Geometry: final body of the model. Coordinates: model frame, mm. A direction names the side the tool comes from. Coordinates: 2 decimals unless noted, no trailing zeros. Answer as a JSON object with one key per item and string values. Group by question number.
Item 1: Set-up query: faces 1 (the cylindrical face through (2.75, -62.44, -10.51)), 2 (the flat face through (-46, 37, -7.3)). Return all of +Z, -Z, +X, -X, +Y, -Y with unobstructed straight access to the full face (end or side cutting, diameter ignored); none if empty.
Item 2: Line query: line 1 along Z through (x, y) = (52.5, 26); line 2 along X through (y, z) = (0, -2); line 3 along X through (y, z) = (0, 0). Output: solid intervals per line, ascending. Write a range as from..to.
Item 3: Mould query, pull axis Z, two halves, no side actions, for faces 3 (the cylindrical face through (-57.11, -12.68, -4.22)), 4 (the cylindrical face through (-57.11, -12.68, 4.18)), 5 (the flat face through (-32, -47, -11.5)), 6 (the cylindrical face through (2.75, -62.44, 6.29)). Classes: pulls with the +Z half, pulls with the -Z half, needs draft (parallel to the pull), parting line crosses it, or undercut.
Item 4: First-contact query: pin 1 Ø1 at (y, z) = (-31.5, 6.5) entering from -X; pin 2 Ø5 at (y, z) = (4, 4.5) entering from -X; pin 3 Ø6 at (x, z) = (19, 0) entering from +Y. Flat tips, straight axial feed; report the tip coordinate or a pass-through.
```python
from build123d import *


with BuildPart() as part:
    # Schizzo2 → Rivoluzione1 (revolve)
    with BuildSketch(Plane(origin=(0, 0, 0), x_dir=(0, 0, -1), z_dir=(1, 0, 0))):
        Polygon((0, 56.5), (-10.5, 56.5), (-11.5, 57.5), (-11.5, 62.5), (-9.5, 62.5), (-9.5, 58.5), (-7.3, 58.5), (-7.3, 62.5), (-5.3, 62.5), (-5.3, 58.5), (-3.1, 58.5), (-3.1, 62.5), (-1.1, 62.5), (-1.1, 58.5), (1.1, 58.5), (1.1, 62.5), (3.1, 62.5), (3.1, 58.5), (5.3, 58.5), (5.3, 62.5), (7.3, 62.5), (7.3, 58.5), (9.5, 58.5), (9.5, 62.5), (11.5, 62.5), (11.5, 56.5), align=None)
    revolve(axis=Axis((0, 0, 0), (0, 0, -1)))


solid = part.part
```
Checks:
{
 "1": {"face 1": "+Z, -Z", "face 2": "none"},
 "2": {"line 1": "-11.5..-9.5, -7.3..-5.3, -3.1..-1.1, 1.1..3.1, 5.3..7.3, 9.5..11.5", "line 2": "-62.5..-56.5, 56.5..62.5", "line 3": "-58.5..-56.5, 56.5..58.5"},
 "3": {"face 3": "undercut", "face 4": "undercut", "face 5": "pulls with the -Z half", "face 6": "needs draft"},
 "4": {"pin 1": "x = -54.27", "pin 2": "x = -62.48", "pin 3": "y = 60.36"}
}
